```python
from build123d import *

# Parameters (mm, degrees)
BOSS_EXTRUDE1_DEPTH = 5
SKETCH3_R           = 1.5
SKETCH3_R_2         = 10.9982
CUT_EXTRUDE1_DEPTH  = 5
SKETCH5_W           = 5
SKETCH5_H           = 5
BOSS_EXTRUDE2_DEPTH = 18.62
SKETCH6_W           = 5
SKETCH6_H           = 18.62
BOSS_EXTRUDE3_DEPTH = 20
CUT_EXTRUDE2_REACH  = 62.095
SKETCH7_R           = 2.75
FILLET1_R           = 3


with BuildPart() as part:
    # Sketch1 → Boss-Extrude1 (new body)
    with BuildSketch(Plane(origin=(0, 0, 0), x_dir=(1, 0, 0), z_dir=(0, 1, 0))):
        with BuildLine():
            Line((-13.883812864, -21.209), (-21.209, -21.209))
            Line((-21.209, -21.209), (-21.209, -13.883812864))
            Line((-21.209, -13.883812864), (-21.209, 13.883812864))
            Line((-21.209, 13.883812864), (-21.209, 21.209))
            Line((-21.209, 21.209), (-13.883812864, 21.209))
            Line((-13.883812864, 21.209), (13.883812864, 21.209))
            ThreePointArc((13.883812864, 21.209), (17.924591218, 17.924591218), (21.209, 13.883812864))
            Line((21.209, 13.883812864), (21.209, -13.883812864))
            ThreePointArc((21.209, -13.883812864), (17.924591218, -17.924591218), (13.883812864, -21.209))
            Line((13.883812864, -21.209), (-13.883812864, -21.209))
        make_face()
    extrude(amount=BOSS_EXTRUDE1_DEPTH)

    # Sketch3 → Cut-Extrude1 (cut)
    with BuildSketch(Plane(origin=(0, 0, 0), x_dir=(1, 0, 0), z_dir=(0, 1, 0))):
        with Locations(Location((15.494, -15.494, 0), (0, 0, 270))):
            Circle(SKETCH3_R)
        with Locations(Location((15.494, 15.494, 0), (0, 0, 270))):
            Circle(SKETCH3_R)
        with Locations(Location((-15.494, -15.494, 0), (0, 0, 270))):
            Circle(SKETCH3_R)
        with Locations(Location((-15.494, 15.494, 0), (0, 0, 270))):
            Circle(SKETCH3_R)
        with Locations(Location((0, 0, 0), (0, 0, 270))):
            Circle(SKETCH3_R_2)
    extrude(amount=CUT_EXTRUDE1_DEPTH, mode=Mode.SUBTRACT)

    # Sketch5 → Boss-Extrude2 (add)
    with BuildSketch(Plane.XY.offset(21.209)):
        with Locations((-18.709, 2.5)):
            Rectangle(SKETCH5_W, SKETCH5_H)
    boss_extrude2 = extrude(amount=BOSS_EXTRUDE2_DEPTH)

    # Sketch6 → Boss-Extrude3 (add)
    with BuildSketch(Plane(origin=(0, 5, 0), x_dir=(1, 0, 0), z_dir=(0, 1, 0))):
        with Locations((-18.709, -30.519)):
            Rectangle(SKETCH6_W, SKETCH6_H)
    boss_extrude3 = extrude(amount=BOSS_EXTRUDE3_DEPTH)

    # Sketch7 → Cut-Extrude2 (cut, up to next)
    with BuildSketch(Plane(origin=(-16.209, 0, 0), x_dir=(0, 0, -1), z_dir=(1, 0, 0)), mode=Mode.PRIVATE) as cut_extrude2_sk1:
        with Locations((-32.829, 16.5)):
            Circle(SKETCH7_R)
    cut_extrude2_tool1 = extrude(cut_extrude2_sk1.sketch, amount=-CUT_EXTRUDE2_REACH, mode=Mode.PRIVATE) & part.part
    cut_extrude2 = cut_extrude2_tool1.solids().sort_by_distance((-16.209, 16.5, 32.829))[0]
    add(cut_extrude2, mode=Mode.SUBTRACT)

    # Mirror3: Boss-Extrude2, Boss-Extrude3, Cut-Extrude2 across plane
    add(boss_extrude2.mirror(Plane(origin=(0, 0, 0), x_dir=(1, 0, 0), z_dir=(0, 0, -1))))
    add(boss_extrude3.mirror(Plane(origin=(0, 0, 0), x_dir=(1, 0, 0), z_dir=(0, 0, -1))))
    add(cut_extrude2.mirror(Plane(origin=(0, 0, 0), x_dir=(1, 0, 0), z_dir=(0, 0, -1))), mode=Mode.SUBTRACT)

    # Fillet1
    fillet1_edges = [part.edges().sort_by_distance(p)[0] for p in [
        (-16.209, 2.5, 21.209),
        (-18.709, 0, 39.829),
        (-18.709, 0, -39.829),
        (-18.709, 25, 39.829),
        (-18.709, 25, -39.829),
        (-16.209, 2.5, -21.209),
        (-18.709, 25, -21.209),
        (-18.709, 25, 21.209),
    ]]
    fillet(fillet1_edges, radius=FILLET1_R)


solid = part.part
```
Here's how the part is built. I have some questions about the finished solid (model axes, mm). A direction names the side the tool comes from. Round coordinates to 2 decimals unless told otherwise and drop trailing zeros. Order: outer loops, then holes, each group sorted by start corner. A loop starts at its lowest first (then second) coordinate and runs counter-clockwise, first axis right, second up. Notation, with made-up numbers: (14.25, -32.75) -> (65.25, -32.75) arc R20 ccw to (65.25, 1.25) -> close; hole circle Ø5 at (53.25, 53). An arc over 180 degrees is marked (long way). Use a Markdown table: item, result. Add a question column.
(1) If we mould it in two halves opening along Z, with no side actions, what happens to faces 1 (the face through (-15.428, 2.465, -16.993)), 2 (the face through (-16.209, 12, -31)), 3 (the face through (-6.69, 2.46, -8.73)), 4 (the face through (-18.67, 0.9, -38.97))? For each: released by +Z, released by -Z, zero draft, split by the parting line, or undercut.
(2) For faces 5 (the face through (-18.674, 24.145, 22.111)), 6 (the face through (0, 2, -21.209)), 7 (the face through (-19, 12, -39.829)), which set-ups out of +Z, -Z, +X, -X, +Y, -Y let a thin tool reach every point of the face, with its end or its side?
(3) Suppose I cut it at C-C, the plane z = 0. Please give me the cut outline in (x, y), and give its area (3 significant figures).
(4) Suppose I cut it at A-A, the plane x = 0. Please give me the cut outline in (y, z), and give its area (3 significant figures).
(5) Suppose I cut it at B-B, the plane y = 16.5. Please give me the cut outline in (x, z), and give its area (3 significant figures).
(6) Suppose I cut it at D-D, the plane z = -29. Please give me the cut outline in (x, y).
(7) For pin 1 Ø1.5 at (x, z) = (-16.5, -19) entering from -Y; pin 2 Ø9.5 at (y, z) = (11.5, 32.5) entering from +X; pin 3 Ø4 at (x, y) = (1.5, 1.5) entering from -Z; pin 4 Ø1.5 at (x, y) = (-2, 3) entering from +Z, each with a flat end and sliding along its axis, tell me the tip position at first contact or that it passes through.
(8) I need wall thicknesses on line 1 along Y through (x, z) = (-15, -8); line 2 along X through (y, z) = (23.25, 30); line 3 along X through (y, z) = (1.75, -2.5). Which ranges of each line are inside material? Lowest first, please.
Verdict:
| question | item | result |
|---|---|---|
| 1 | face 1 | undercut |
| 1 | face 2 | zero draft |
| 1 | face 3 | undercut |
| 1 | face 4 | released by -Z |
| 2 | face 5 | +X, -X, +Y |
| 2 | face 6 | -Z, +X, +Y, -Y |
| 2 | face 7 | -Z, +X, -X, +Y, -Y |
| 3 | outline | (-21.21, 0) -> (-11, 0) -> (-11, 5) -> (-21.21, 5) -> close; (11, 0) -> (21.21, 0) -> (21.21, 5) -> (11, 5) -> close |
| 3 | area | 102 mm2 |
| 4 | outline | (0, -21.21) -> (5, -21.21) -> (5, -11) -> (0, -11) -> close; (0, 11) -> (5, 11) -> (5, 21.21) -> (0, 21.21) -> close |
| 4 | area | 102 mm2 |
| 5 | outline | (-21.21, -39.83) -> (-16.21, -39.83) -> (-16.21, -35.58) -> (-21.21, -35.58) -> close; (-21.21, -30.08) -> (-16.21, -30.08) -> (-16.21, -21.21) -> (-21.21, -21.21) -> close; (-21.21, 21.21) -> (-16.21, 21.21) -> (-16.21, 30.08) -> (-21.21, 30.08) -> close; (-21.21, 35.58) -> (-16.21, 35.58) -> (-16.21, 39.83) -> (-21.21, 39.83) -> close |
| 5 | area | 131 mm2 |
| 6 | outline | (-21.21, 0) -> (-16.21, 0) -> (-16.21, 25) -> (-21.21, 25) -> close |
| 7 | pin 1 | y = 0 |
| 7 | pin 2 | x = -16.21 |
| 7 | pin 3 | z = -21.21 |
| 7 | pin 4 | z = 21.21 |
| 8 | line 1 | 0 to 5 |
| 8 | line 2 | -21.21 to -16.21 |
| 8 | line 3 | -21.21 to -10.71, 10.71 to 21.21 |
